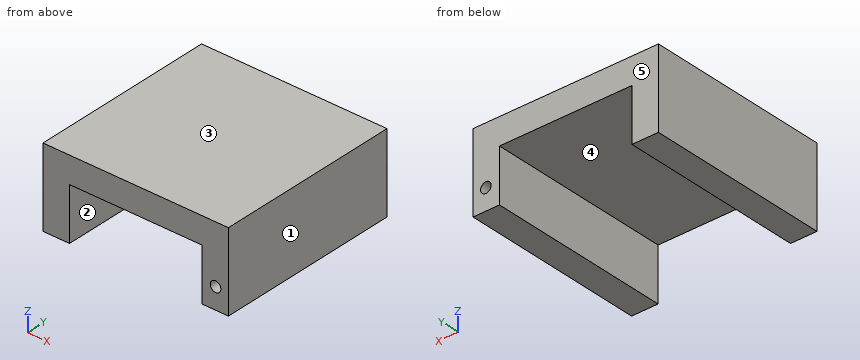
from build123d import *

# Parameters (mm, degrees)
F0_R     = 2.54
F1_DEPTH = 88.9


with BuildPart() as f1:
    # F0 (on Front) → F1 (new body)
    with BuildSketch(Plane.XZ):
        Polygon((-88.9, -38.0440002276), (-76.2, -38.0440002276), (-76.2, -12.6440002276), (-12.7, -12.6440002276), (-12.7, -38.0440002276), (0, -38.0440002276), (0, 0.0559997724), (-88.9, 0.0559997724), (-88.9, -12.6440002276), align=None)
        with Locations((-6.1765108258, -27.8850197792)):
            Circle(F0_R, mode=Mode.SUBTRACT)
    extrude(amount=F1_DEPTH)


with BuildPart() as f1b:
    # F0 (on Front) → F1, piece 2 (new body)
    with BuildSketch(Plane.XZ):
        with Locations((-59.0428002179, -29.2415227741)):
            Circle(F0_R)
    extrude(amount=F1_DEPTH)


solid = f1.part
Work out the finished part from the listing and answer in its coordinate system (mm). Face numbers are marked on the shaded views. A direction names the side the tool comes from. Round coordinates to 2 decimals unless told otherwise and drop trailing zeros. Write each loop counter-clockwise with the first axis right and the second up, starting at its lowest first coordinate (ties: lowest second). Pieces come first, ordered by that corner, then holes.
1) Given pin 1 Ø6 at (x, y) = (-16, -14.5) entering from -Z, flat-ended and moving along its own axis, determine where the tip first touches the part or whether it passes through.
2) A cutting plane is placed at D-D (x = -51.5). Give the vertices of the cut face in (y, z).
3) Straight lines are drawn through the part: line 1 (X direction, y = -35.5, z = -13.5); line 2 (X direction, y = -41, z = -28.5); line 3 (X direction, y = -81.5, z = -29.5). For each, find the intervals that lie inside material, in ascending order.
4) A cutting plane is placed at B-B (x = -6.5). Give the vertices of the cut face in (y, z).
5) A tool of negligible diameter and unlimited length cuts with its end or side. For the marked faces 4 and 5, from which of +Z, -Z, +X, -X, +Y, -Y can it reach the whole face along a straight path? Write none if from no direction.
6) The mould has two halves that part along X. Classify the marked faces 1, 2 and 3: pulls with the +X half, pulls with the -X half, needs draft (parallel to the pull), parting line crosses it, or undercut.
7) A cutting plane is placed at C-C (y = -59.5). Give the vertices of the cut face in (x, z), plus the area to 3 significant figures.
8) A cutting plane is placed at A-A (z = -18). Give the vertices of the cut face in (x, y).
Completed:
1. pin 1: stops at z = -12.64
2. outline: (-88.9, -12.64) - (0, -12.64) - (0, 0.06) - (-88.9, 0.06) - close
3. line 1: x = -88.9 to -76.2, -12.7 to 0
3. line 2: x = -88.9 to -76.2, -12.7 to -8.64, -3.71 to 0
3. line 3: x = -88.9 to -76.2, -12.7 to -8.14, -4.22 to 0
4. outline: (-88.9, -38.04) - (0, -38.04) - (0, -30.4) - (-88.9, -30.4) - close; (-88.9, -25.37) - (0, -25.37) - (0, 0.06) - (-88.9, 0.06) - close
5. face 4: -Z, +Y, -Y
5. face 5: +Z, -Z, +X, -X, +Y
6. face 1: pulls with the +X half
6. face 2: undercut
6. face 3: needs draft
7. outline: (-88.9, -38.04) - (-76.2, -38.04) - (-76.2, -12.64) - (-12.7, -12.64) - (-12.7, -38.04) - (0, -38.04) - (0, 0.06) - (-88.9, 0.06) - close; hole circle Ø5.08 at (-6.18, -27.89)
7. area: 1,750 mm2
8. outline: (-88.9, -88.9) - (-76.2, -88.9) - (-76.2, 0) - (-88.9, 0) - close; (-12.7, -88.9) - (0, -88.9) - (0, 0) - (-12.7, 0) - close
